Input: part model. Units: mm. Frame: model coordinates. A direction names the side the tool comes from. Coordinates: 2 decimals unless noted, no trailing zeros. Loops run counter-clockwise (first coordinate to the right, second up) from the corner with the lowest first, then second, coordinate; pieces in that order, holes last. Notation, with made-up numbers: (3.5, -28.75) - (34.5, -28.75) arc R13 ccw to (34.5, -18.75) - close; hole circle Ø4 at (52.5, 66.25). An arc over 180 degrees is marked (long way). Use a Markdown table: item, result. Add a question column.
1. Ray query, L1, parallel to X at y = 1, z = -70; L2, parallel to X at y = 5, z = -130 (3 decimals); L3, parallel to Z at x = 149, y = 1. Return the intervals inside material, ascending. Write a range as [from, to].
2. Section query B-B on y = 1.75. Return the cut outline in (x, z) (3 decimals), then the cut area to 3 significant figures.
3. Draft query along X for faces 3 (the face through (185.42, 3, -120)), 4 (the face through (135, 3, -110.077)), 5 (the face through (134, 3, -184.15)). Return one class per face: released by +X, released by -X, zero draft, split by the parting line, or undercut.
4. Contact query for a flat-ended pin moving along its axis: P1, Ø3.5, axis at x = 134.62, z = -69.85, coming from the +Y side. Output: stop coordinate, or through.
5. Section query A-A on z = -171.45. Return the cut outline in (x, y), then the cut area to 3 significant figures.
6. Access query for faces 1 (the face through (134, 0, -107)), 2 (the face through (113.665, 3, -121)). Directions: +Z, -Z, +X, -X, +Y, -Y. A direction counts if a zero-diameter tool reaches every point of the face in a straight line with its end or side. Return the directions, or none.
```python
from build123d import *

# Parameters (mm, degrees)
SKETCH1_W           = 101.6
SKETCH1_H           = 127
BOSS_EXTRUDE1_DEPTH = 6.35
SKETCH2_R           = 2.032
SKETCH2_W           = 43.18
SKETCH2_H           = 21.1455
CUT_EXTRUDE1_DEPTH  = 7.35
SKETCH7_R           = 1.5
CUT_EXTRUDE2_DEPTH  = 7.35


with BuildPart() as part:
    # Sketch1 → Boss-Extrude1 (new body)
    with BuildSketch(Plane(origin=(0, 0, 0), x_dir=(1, 0, 0), z_dir=(0, 1, 0))):
        with Locations((134.62, 120.65)):
            Rectangle(SKETCH1_W, SKETCH1_H)
    extrude(amount=BOSS_EXTRUDE1_DEPTH)

    # Sketch2 → Cut-Extrude1 (cut, through all)
    with BuildSketch(Plane(origin=(0, 6.35, 0), x_dir=(1, 0, 0), z_dir=(0, 1, 0))):
        with Locations((109.855, 116.99875)):
            Circle(SKETCH2_R)
        with Locations((109.855, 125.63475)):
            Circle(SKETCH2_R)
        with Locations((160.655, 125.63475)):
            Circle(SKETCH2_R)
        with Locations((160.655, 116.99875)):
            Circle(SKETCH2_R)
        with Locations((135.255, 120.65)):
            Rectangle(SKETCH2_W, SKETCH2_H)
    extrude(amount=-CUT_EXTRUDE1_DEPTH, mode=Mode.SUBTRACT)

    # Sketch7 → Cut-Extrude2 (cut, through all)
    with BuildSketch(Plane(origin=(0, 6.35, 0), x_dir=(1, 0, 0), z_dir=(0, 1, 0))):
        with Locations((134.62, 171.45)):
            Circle(SKETCH7_R)
        with Locations((134.62, 69.85)):
            Circle(SKETCH7_R)
    extrude(amount=-CUT_EXTRUDE2_DEPTH, mode=Mode.SUBTRACT)


solid = part.part
```
Resolved:
| question | item | result |
|---|---|---|
| 1 | L1 | [83.82, 133.13], [136.11, 185.42] |
| 1 | L2 | [83.82, 113.665], [156.845, 185.42] |
| 1 | L3 | [-184.15, -131.22], [-110.08, -57.15] |
| 2 | outline | (83.82, -184.15) - (185.42, -184.15) - (185.42, -57.15) - (83.82, -57.15) - close; hole circle Ø4.064 at (109.855, -125.635); hole circle Ø4.064 at (109.855, -116.999); hole (113.665, -131.223) - (156.845, -131.223) - (156.845, -110.077) - (113.665, -110.077) - close; hole circle Ø3 at (134.62, -171.45); hole circle Ø3 at (134.62, -69.85); hole circle Ø4.064 at (160.655, -125.635); hole circle Ø4.064 at (160.655, -116.999) |
| 2 | area | 11,900 mm² |
| 3 | face 3 | released by +X |
| 3 | face 4 | undercut |
| 3 | face 5 | zero draft |
| 4 | P1 | y = 6.35 |
| 5 | outline | (83.82, 0) - (133.12, 0) - (133.12, 6.35) - (83.82, 6.35) - close; (136.12, 0) - (185.42, 0) - (185.42, 6.35) - (136.12, 6.35) - close |
| 5 | area | 626 mm² |
| 6 | face 1 | +Z, -Z, +X, -X, -Y |
| 6 | face 2 | +Y, -Y |
